from build123d import *

# Parameters (mm, degrees)
HOLE1_D           = 6.4389
HOLE1_DEPTH       = 38.8874
HOLE1_CSINK_D     = 7.9629
HOLE1_CSINK_ANGLE = 90


with BuildPart() as part:
    # Sketch1 → Revolve1 (revolve)
    with BuildSketch(Plane.XY):
        with BuildLine():
            Line((0, 0), (0, 7.09803))
            Line((0, 7.09803), (0.83947, 7.9375))
            Line((0.83947, 7.9375), (6.469412072, 7.9375))
            Line((6.469412072, 7.9375), (7.30937001, 7.098844511))
            ThreePointArc((7.30937001, 7.098844511), (7.597613092, 6.906489173), (7.9375, 6.83895))
            Line((7.9375, 6.83895), (9.2202, 6.83895))
            ThreePointArc((9.2202, 6.83895), (9.848817928, 7.099332072), (10.1092, 7.72795))
            Line((10.1092, 7.72795), (10.1092, 7.90575))
            Line((10.1092, 7.90575), (12.4968, 7.90575))
            Line((12.4968, 7.90575), (12.4968, 0))
            Line((12.4968, 0), (0, 0))
        make_face()
    revolve(axis=Axis((12.4968, 0, 0), (-1, 0, 0)))

    # Sketch2 → Revolve2 (revolve)
    with BuildSketch(Plane.XY):
        Polygon((12.4968, 0), (12.4968, 10.9982), (13.2588, 11.7602), (32.5374, 11.7602), (32.5374, 10.48385), (33.2994, 10.48385), (34.0614, 11.24585), (38.1254, 11.24585), (38.8874, 10.48385), (38.8874, 0), align=None)
    revolve(axis=Axis((38.8874, 0, 0), (-1, 0, 0)))

    # Hole1
    with Locations(Plane.ZY):
        with Locations((0, 0)):
            CounterSinkHole(HOLE1_D / 2, HOLE1_CSINK_D / 2, depth=HOLE1_DEPTH, counter_sink_angle=HOLE1_CSINK_ANGLE)

    # Sketch5 → Cut-Revolve1 (revolve, cut)
    with BuildSketch(Plane(origin=(0, 0, 0), x_dir=(1, 0, 0), z_dir=(0, 1, 0))):
        Polygon((24.6126, 0), (27.7876, 0), (27.7876, -2.713616984), (29.214183016, -4.1402), (29.452075925, -11.7602), (24.6126, -11.7602), align=None)
    revolve(axis=Axis((24.6126, 0, 11.7602), (0, 0, -1)), mode=Mode.SUBTRACT)

    # Sketch6 → Revolve3 (revolve)
    with BuildSketch(Plane.XY):
        with BuildLine():
            Line((32.5374, 10.22985), (33.2994, 10.22985))
            Line((33.2994, 10.22985), (33.2994, 10.48385))
            Line((33.2994, 10.48385), (32.9184, 10.48385))
            Line((32.9184, 10.48385), (32.659887194, 10.742362806))
            ThreePointArc((32.659887194, 10.742362806), (32.622689755, 10.832165367), (32.659887194, 10.921967928))
            Line((32.659887194, 10.921967928), (33.41395107, 11.676031804))
            Line((33.41395107, 11.676031804), (33.41395107, 11.7602))
            Line((33.41395107, 11.7602), (33.21075107, 11.7602))
            Line((33.21075107, 11.7602), (32.5374, 11.08684893))
            Line((32.5374, 11.08684893), (32.5374, 10.22985))
        make_face()
    revolve(axis=Axis((33.2994, 0, 0), (-1, 0, 0)))


solid = part.part
Design review of the part built by this model. Coordinates are the model's own, in mm. A direction names the side the tool comes from. Coordinates: 2 decimals unless noted, no trailing zeros. Order: outer loops, then holes, each group sorted by start corner. A loop starts at its lowest first (then second) coordinate and runs counter-clockwise, first axis right, second up. Notation, with made-up numbers: (29, 74) - (60, 74) arc R26 ccw to (60, 92) - close; hole circle Ø6 at (66.25, -22). An arc over 180 degrees is marked (long way). Put each result on its own line as item: value.
1) The part is to be moulded in two halves that separate along Y. For faces 1 (the face through (36.12, 6.05, -9.48)), 2 (the face through (24.657, -3.175, 1.881)), 3 (the face through (0, -3, 3)), say which applies: released by +Y, released by -Y, zero draft, split by the parting line, or undercut.
Response values:
face 1: split by the parting line
face 2: undercut
face 3: zero draft
2) Take a section at C-C, the plane x = 32. Give the boundary of the cut face in (y, z).
Response values:
outline: circle Ø23.52 at (0, 0); hole circle Ø6.44 at (0, 0)
3) Wall thickness on L1, parallel to Z at x = 11.5, y = 0; L2, parallel to Y at x = 24.5, z = 0; L3, parallel to X at y = 9.25, z = -4.75: over which ranges is each line inside the solid? List them lowest first. Write a range as from..to.
Response values:
L1: z = -7.91..-3.22, 3.22..7.91
L2: y = -11.76..-3.22, 3.22..11.76
L3: x = 12.5..38.89
4) Tool access review of faces 4 (the face through (38.887, -2.5, -2.5)), 5 (the face through (24.568, 3.175, 1.881)), 6 (the face through (33.11, 10, -3.15)): name each direction out of +Z, -Z, +X, -X, +Y, -Y from which nothing blocks a thin tool from reaching the whole face with its end or side.
Response values:
face 4: +Z, -Z, +X, +Y, -Y
face 5: +Z
face 6: none
5) Take a section at B-B, the plane y = 0. Count the separate pieces of the cut face and the enclosed holes in it, and give its area (3 significant figures).
Response values:
separate pieces: 3
enclosed holes: 0
area: 472 mm²
6) Insertion check: P1, Ø12, axis at x = 21, y = 8.5, coming from the +Z side; P2, Ø2, axis at x = 17, z = -8, coming from the -Y side; P3, Ø5, axis at x = 20.5, y = -8, coming from the -Z side. Each pin has a flat end and moves straight along its axis. Give the tip position at first contact, or say it passes through.
Response values:
P1: stops at z = 11.49
P2: stops at y = -9.45
P3: stops at z = -10.39
7) Take a section at A-A, the plane x = 36. Give the boundary of the cut face in (y, z), and give its area (3 significant figures).
Response values:
outline: circle Ø22.49 at (0, 0); hole circle Ø6.44 at (0, 0)
area: 365 mm²
